from build123d import *

# Parameters (mm, degrees)
BOSS_EXTRUDE1_DEPTH = 550
SKETCH2_R           = 3
CUT_EXTRUDE2_DEPTH  = 200
SKETCH3_W           = 47.285738773
SKETCH3_H           = 54.700142613
CUT_EXTRUDE3_DEPTH  = 6


with BuildPart() as part:
    # Sketch1 → Boss-Extrude1 (new body)
    with BuildSketch(Plane.XY):
        Polygon((25.5, 43), (25.5, 45), (40, 45), (40, 0), (0, 0), (0, 45), (14.5, 45), (14.5, 43), (9.595309941, 43), (7.5, 43), (7.5, 35), (32.5, 35), (32.5, 43), align=None)
        Polygon((33.5, 44), (33.5, 34), (6.5, 34), (6.5, 44), (1, 44), (1, 1), (39, 1), (39, 44), align=None, mode=Mode.SUBTRACT)
    extrude(amount=BOSS_EXTRUDE1_DEPTH)

    # Sketch2 → Cut-Extrude2 (cut)
    with BuildSketch(Plane(origin=(0, 35, 0), x_dir=(1, 0, 0), z_dir=(0, 1, 0))):
        with Locations(Location((20, -40, 0), (0, 0, 180))):
            Circle(SKETCH2_R)
        with Locations(Location((20, -510, 0), (0, 0, 180))):
            Circle(SKETCH2_R)
    extrude(amount=-CUT_EXTRUDE2_DEPTH, mode=Mode.SUBTRACT)

    # Sketch3 → Cut-Extrude3 (cut)
    with BuildSketch(Plane(origin=(0, 0, 0), x_dir=(-1, 0, 0), z_dir=(0, 0, -1))):
        with Locations((-18.970719089, 19.421785252)):
            Rectangle(SKETCH3_W, SKETCH3_H)
    extrude(amount=-CUT_EXTRUDE3_DEPTH, mode=Mode.SUBTRACT)


solid = part.part
Model file for the job. Use its own axes, mm. A direction names the side the tool comes from. Give positions to 0.01 mm unless a question says otherwise; leave off trailing zeros. Write each loop counter-clockwise with the first axis right and the second up, starting at its lowest first coordinate (ties: lowest second). Pieces come first, ordered by that corner, then holes. Notation, with made-up numbers: M -1,11.25 L 11,11.25 A27 ccw 11,31.25 Z; hole C -4,22.25 d8. An arc over 180 degrees is marked long. One line per item, written item: value. Start each with the question number.
Q1. Saw through at B-B, the plane y = 29.5. Write the cut outline in (x, z).
Q2. Probe probe 1 along X at (y, z) = (42, 162); probe 2 along Y at (x, z) = (13.5, 277.5); probe 3 along Z at (x, y) = (20, 34.8). List the from-to ranges inside material, lowest first. Write a range as [from, to].
Q3. Saw through at A-A, the plane z = 250.5. Write the cut outline in (x, y).
Q4. 3-axis set-ups, long thin cutter, end or side, ignore diameter. For faces 4 (the flat face through (20.1, 34.3, 550)), 5 (the flat face through (20, 35, 274)): which of +Z, -Z, +X, -X, +Y, -Y reach the whole face in a straight line?
Q5. Drop a flat-ended pin along its axis: pin 1 Ø5 at (x, z) = (20, 40) entering from -Y. Give the stop position or say it passes through.
Q6. Two-plate mould, pull along Y, no slides. Class faces 1 (the flat face through (33, 45, 274)), 2 (the flat face through (39, 22, 274)), 3 (the flat face through (0, 22, 274)): +Y half, -Y half, draft (parallel to the pull), parting line (faces both ways), or undercut.
Output values:
1. outline: M 0,6 L 1,6 L 1,550 L 0,550 Z; M 39,6 L 40,6 L 40,550 L 39,550 Z
2. probe 1: x = [0, 1], [6.5, 7.5], [32.5, 33.5], [39, 40]
2. probe 2: y = [0, 1], [34, 35], [43, 45]
2. probe 3: z = [6, 37], [43, 507], [513, 550]
3. outline: M 0,0 L 40,0 L 40,45 L 25.5,45 L 25.5,43 L 32.5,43 L 32.5,35 L 7.5,35 L 7.5,43 L 14.5,43 L 14.5,45 L 0,45 Z; hole M 1,1 L 39,1 L 39,44 L 33.5,44 L 33.5,34 L 6.5,34 L 6.5,44 L 1,44 Z
4. face 4: +Z, +X, -X, +Y, -Y
4. face 5: +Z, -Z
5. pin 1: passes through
6. face 1: +Y half
6. face 2: undercut
6. face 3: draft
